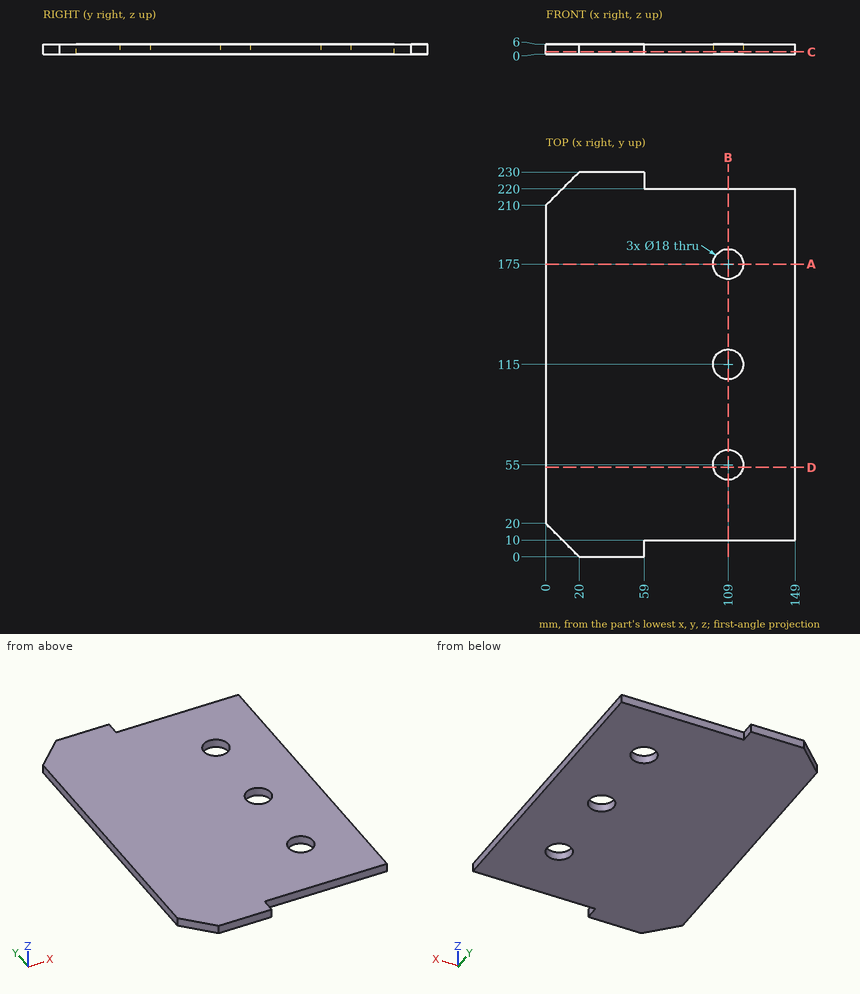
Can you work these out from the drawing? Everything is in mm from the part's minimum corner. Round coordinates to 2 decimals unless told otherwise and drop trailing zeros. Loops run counter-clockwise (first coordinate to the right, second up) from the corner with the lowest first, then second, coordinate; pieces in that order, holes last. Notation, with made-up numbers: (31.25, 78) - (60.25, 78) arc R23 cw to (60.25, 91) - close; hole circle Ø3 at (2.5, -4). An arc over 180 degrees is marked (long way). Answer in a Markdown table with one row per item. Add a question column.
Q1. For pin 1 Ø20.5 at (x, y) = (109, 115) entering from -Z; pin 2 Ø1.8 at (x, z) = (90, 3) entering from -Y; pin 3 Ø3 at (y, z) = (223, 2.5) entering from +X, each with a flat end and sliding along its axis, tell me the tip position at first contact or that it passes through.
Q2. I need wall thicknesses on L1, parallel to Y at x = 109, z = 3; L2, parallel to X at y = 115, z = 2.25; L3, parallel to Y at x = 126.5, z = 2.9. Which ranges of each line are inside material? Lowest first, please.
Q3. I want a section at A-A on y = 175. List the corners of the cut face in (x, z) for me, and give its area (3 significant figures).
Q4. I want a section at B-B on x = 109. List the corners of the cut face in (y, z) for me.
Q5. I want a section at C-C on z = 1.25. List the corners of the cut face in (x, y) for me, and give its area (3 significant figures).
Q6. I want a section at D-D on y = 53.5. List the corners of the cut face in (x, z) for me, and give its area (3 significant figures).
A:
| question | item | result |
|---|---|---|
| 1 | pin 1 | z = 0 |
| 1 | pin 2 | y = 10 |
| 1 | pin 3 | x = 59 |
| 2 | L1 | 10 to 46, 64 to 106, 124 to 166, 184 to 220 |
| 2 | L2 | 0 to 100, 118 to 149 |
| 2 | L3 | 10 to 220 |
| 3 | outline | (0, 0) - (100, 0) - (100, 6) - (0, 6) - close; (118, 0) - (149, 0) - (149, 6) - (118, 6) - close |
| 3 | area | 786 mm^2 |
| 4 | outline | (10, 0) - (46, 0) - (46, 6) - (10, 6) - close; (64, 0) - (106, 0) - (106, 6) - (64, 6) - close; (124, 0) - (166, 0) - (166, 6) - (124, 6) - close; (184, 0) - (220, 0) - (220, 6) - (184, 6) - close |
| 5 | outline | (0, 20) - (20, 0) - (59, 0) - (59, 10) - (149, 10) - (149, 220) - (59, 220) - (59, 230) - (20, 230) - (0, 210) - close; hole circle Ø18 at (109, 55); hole circle Ø18 at (109, 115); hole circle Ø18 at (109, 175) |
| 5 | area | 31,300 mm^2 |
| 6 | outline | (0, 0) - (100.13, 0) - (100.13, 6) - (0, 6) - close; (117.87, 0) - (149, 0) - (149, 6) - (117.87, 6) - close |
| 6 | area | 788 mm^2 |
